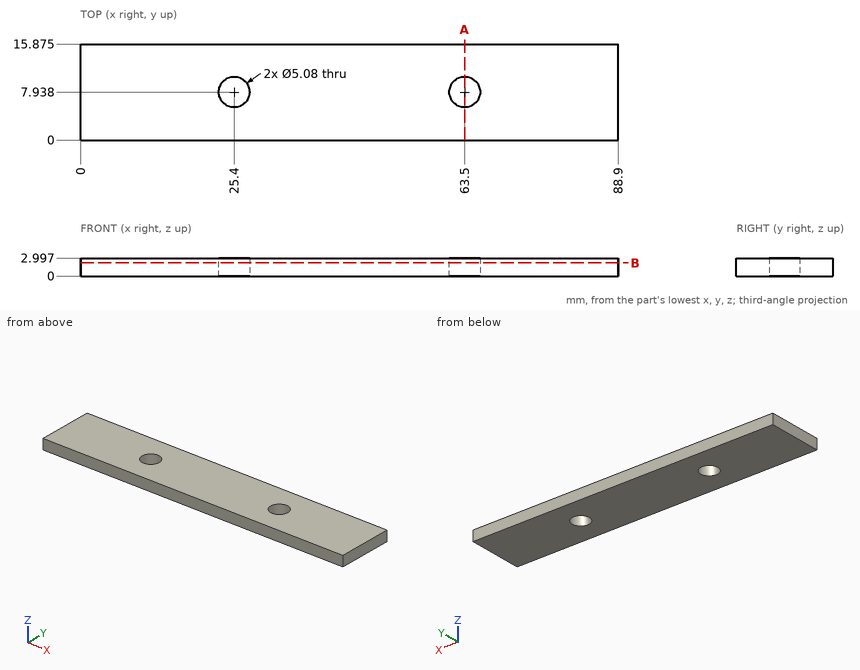
The drawing under review shows one solid part. Ordinate dimensions are in mm from its lowest x, y, z. Round coordinates to 2 decimals unless told otherwise and drop trailing zeros. Loops run counter-clockwise (first coordinate to the right, second up) from the corner with the lowest first, then second, coordinate; pieces in that order, holes last. Notation, with made-up numbers: M -37.5,66.5 L -0.5,66.5 A20 ccw -0.5,100.5 Z; hole C 89,-39.75 d8. An arc over 180 degrees is marked long. Answer as CSV lines item,"result". Start each with the question number.
Item 1: Insertion check: P1, Ø4.5, axis at x = 63.5, y = 7.94, coming from the -Z side. The pin has a flat end and moves straight along its axis. Give the tip position at first contact, or say it passes through.
Item 2: Consider section B-B (z = 2.2). Write out the cut boundary in (x, y) (1 decimal).
Item 3: Consider section A-A (x = 63.5). Write out the cut boundary in (y, z) (1 decimal).
Item 4: Wall thickness on line 1 (Y direction, x = 25.4, z = 1.55) (1 decimal); line 2 (X direction, y = 7, z = 0.2); line 3 (X direction, y = 7.5, z = 1.5): over which ranges is each line inside the solid? List them lowest first. Write a range as [from, to].
Answer:
1,P1,"passes through"
2,outline,"M 0,0 L 88.9,0 L 88.9,15.9 L 0,15.9 Z; hole C 25.4,7.9 d5.1; hole C 63.5,7.9 d5.1"
3,outline,"M 0,0 L 5.4,0 L 5.4,3 L 0,3 Z; M 10.5,0 L 15.9,0 L 15.9,3 L 10.5,3 Z"
4,line 1,"y = [0, 5.4], [10.5, 15.9]"
4,line 2,"x = [0, 23.04], [27.76, 61.14], [65.86, 88.9]"
4,line 3,"x = [0, 22.9], [27.9, 61], [66, 88.9]"
